Read the model definition and answer for the solid it produces. Units are mm, in the model's axes. A direction names the side the tool comes from. Give positions to 0.01 mm unless a question says otherwise; leave off trailing zeros. Write each loop counter-clockwise with the first axis right and the second up, starting at its lowest first coordinate (ties: lowest second). Pieces come first, ordered by that corner, then holes.
```python
from build123d import *

# Parameters (mm, degrees)
F1_DEPTH = 26
F3_DEPTH = 20
F4_R     = 1


with BuildPart() as f1:
    # F0 (on Top) → F1 (new body)
    with BuildSketch(Plane.XY):
        Polygon((0, 0), (0, -55), (28, -55), (55, -28), (55, 0), align=None)
    extrude(amount=-F1_DEPTH)

    # F2 (on face) → F3 (cut)
    with BuildSketch(Plane(origin=(0, 0, -26), x_dir=(1, 0, 0), z_dir=(0, 0, -1))):
        Polygon((24, 55), (3.8, 55), (3.8, 3.8), (55, 3.8), (55, 24), (24, 24), align=None)
    extrude(amount=-F3_DEPTH, mode=Mode.SUBTRACT)

    # F4
    f4_edges = [f1.edges().sort_by_distance(p)[0] for p in [
        (3.8, -3.8, -16),
        (3.8, -29.4, -6),
        (29.4, -3.8, -6),
        (24, -39.5, -6),
        (39.5, -24, -6),
        (24, -24, -16),
    ]]
    fillet(f4_edges, radius=F4_R)


solid = f1.part
```
Item 1: Determine the mould class of faces 6 (the flat face through (0, -27, -13)), 7 (the flat face through (40, -24, -17)), 8 (the flat face through (28, 0, -13)) for opening direction Y: pulls with the +Y half, pulls with the -Y half, needs draft (parallel to the pull), parting line crosses it, or undercut.
Result set:
face 6: needs draft
face 7: undercut
face 8: pulls with the +Y half
Item 2: Section B-B (x = 38) is taken. Write down the section's boundary in (y, z), and give its area (3 significant figures).
Result set:
outline: (-45, -26) - (-24, -26) - (-24, -7) arc R1 cw to (-23, -6) - (-4.8, -6) arc R1 cw to (-3.8, -7) - (-3.8, -26) - (0, -26) - (0, 0) - (-45, 0) - close
area: 766 mm2
Item 3: Section C-C (z = -17.5) is taken. Write down the section's boundary in (x, y).
Result set:
outline: (0, -55) - (3.8, -55) - (3.8, -4.8) arc R1 cw to (4.8, -3.8) - (55, -3.8) - (55, 0) - (0, 0) - close; (24, -55) - (28, -55) - (55, -28) - (55, -24) - (25, -24) arc R1 ccw to (24, -25) - close
Item 4: Each of these flat-tipped pins is pushed along its axis until it touches: pin 1 Ø6 at (x, y) = (36.5, -12) entering from -Z; pin 2 Ø3 at (y, z) = (-22, -23) entering from +X. Where does it stop, or does it pass through?
Result set:
pin 1: stops at z = -6
pin 2: stops at x = 3.8
Item 5: Find the intervals of material crossed by line 1 along Y through (x, z) = (6.5, -23.5); line 2 along Y through (x, z) = (25, -7); line 3 along Z through (x, y) = (32, -18), in increasing order.
Result set:
line 1: y = -3.8 to 0
line 2: y = -55 to -24, -3.8 to 0
line 3: z = -6 to 0
Item 6: Which of the six approach directions +Z, -Z, +X, -X, +Y, -Y give full straight-line access (tool end or side, diameter ignored) to faces 1 (the flat face through (27, -27, 0)), 2 (the flat face through (24, -19, -6)), 3 (the flat face through (3.8, -30, -17)), 4 (the flat face through (30, -3.8, -17)), 5 (the flat face through (36, -36, -26))?
Result set:
face 1: +Z, +X, -X, +Y, -Y
face 2: -Z
face 3: -Z, -Y
face 4: -Z, +X
face 5: -Z, +X, -X, +Y, -Y
Item 7: Section D-D (z = -2.5) is taken. Write down the section's boundary in (x, y).
Result set:
outline: (0, -55) - (28, -55) - (55, -28) - (55, 0) - (0, 0) - close
Item 8: Section A-A (y = -45) is taken. Write down the section's boundary in (x, z).
Result set:
outline: (0, -26) - (3.8, -26) - (3.8, -7) arc R1 cw to (4.8, -6) - (23, -6) arc R1 cw to (24, -7) - (24, -26) - (38, -26) - (38, 0) - (0, 0) - close
